The model under review builds one solid part; all positions refer to its coordinate system, in mm. A direction names the side the tool comes from. Coordinates: 2 decimals unless noted, no trailing zeros. Write each loop counter-clockwise with the first axis right and the second up, starting at its lowest first coordinate (ties: lowest second). Pieces come first, ordered by that corner, then holes. Notation, with made-up numbers: (50.5, 51) - (95.5, 51) arc R22 cw to (95.5, 68) - close; hole circle Ø7 at (63, 13.25). An arc over 180 degrees is marked (long way). Put each result on its own line as item: value.
from build123d import *

# Parameters (mm, degrees)
SKETCH1_W            = 688.1
SKETCH1_H            = 688.1
SKETCH1_W_2          = 650
SKETCH1_H_2          = 650
BOSS_EXTRUDE1_DEPTH  = 661.9
SKETCH3_W            = 100.2
SKETCH3_H            = 650
SKETCH3_W_2          = 38.6
CUT_EXTRUDE1_DEPTH   = 9.525
SKETCH4_W            = 100.2
SKETCH4_H            = 669.5
SKETCH4_W_2          = 38.6
SKETCH4_H_2          = 669.05
CUT_EXTRUDE3_DEPTH   = 9.525
SKETCH6_W            = 100.2
SKETCH6_H            = 669.5
SKETCH6_W_2          = 38.6
CUT_EXTRUDE4_DEPTH   = 9.525
CUT_EXTRUDE5_DEPTH   = 700
MIRROR6_COPY_1_DEPTH = 700


with BuildPart() as part:
    # Sketch1 → Boss-Extrude1 (new body)
    with BuildSketch(Plane(origin=(0, 0, 0), x_dir=(0, 0, -1), z_dir=(1, 0, 0))):
        with Locations((344.05, 344.05)):
            Rectangle(SKETCH1_W, SKETCH1_H)
        with Locations((344.05, 344.05)):
            Rectangle(SKETCH1_W_2, SKETCH1_H_2, mode=Mode.SUBTRACT)
    extrude(amount=BOSS_EXTRUDE1_DEPTH)

    # Sketch3 → Cut-Extrude1 (cut)
    with BuildSketch(Plane.XY.offset(-669.05)):
        with Locations((171.225, 344.05)):
            Rectangle(SKETCH3_W, SKETCH3_H)
        with Locations((361.75, 344.05)):
            Rectangle(SKETCH3_W_2, SKETCH3_H)
        with Locations((521.475, 344.05)):
            Rectangle(SKETCH3_W_2, SKETCH3_H)
    cut_extrude1 = extrude(amount=-CUT_EXTRUDE1_DEPTH, mode=Mode.SUBTRACT)

    # Mirror2: Cut-Extrude1 across plane
    add(cut_extrude1.mirror(Plane(origin=(0, 0, -344.05), x_dir=(1, 0, 0), z_dir=(0, 0, -1))), mode=Mode.SUBTRACT)

    # Sketch4 → Cut-Extrude3 (cut)
    with BuildSketch(Plane(origin=(0, 19.05, 0), x_dir=(1, 0, 0), z_dir=(0, 1, 0))):
        with Locations((171.225, 343.825)):
            Rectangle(SKETCH4_W, SKETCH4_H)
        with Locations((361.75, 343.825)):
            Rectangle(SKETCH4_W_2, SKETCH4_H)
        with Locations((521.475, 344.05)):
            Rectangle(SKETCH4_W_2, SKETCH4_H_2)
    cut_extrude3 = extrude(amount=-CUT_EXTRUDE3_DEPTH, mode=Mode.SUBTRACT)

    # Mirror4: Cut-Extrude3 across plane
    add(cut_extrude3.mirror(Plane.ZX.offset(344.05)), mode=Mode.SUBTRACT)

    # Sketch6 → Cut-Extrude4 (cut)
    with BuildSketch(Plane(origin=(0, 688.1, 0), x_dir=(1, 0, 0), z_dir=(0, 1, 0))):
        with Locations((171.225, 344.275)):
            Rectangle(SKETCH6_W, SKETCH6_H)
        with Locations((361.75, 343.825)):
            Rectangle(SKETCH6_W_2, SKETCH6_H)
        with Locations((521.475, 343.825)):
            Rectangle(SKETCH6_W_2, SKETCH6_H)
    extrude(amount=-CUT_EXTRUDE4_DEPTH, mode=Mode.SUBTRACT)

    # Sketch7 → Cut-Extrude5 (cut)
    with BuildSketch(Plane.ZY):
        Polygon((-19.05, 39.05), (-9.525, 39.05), (-9.525, 9.525), (-39.05, 9.525), (-39.05, 19.05), (-19.05, 19.05), align=None)
    cut_extrude5 = extrude(amount=-CUT_EXTRUDE5_DEPTH, mode=Mode.SUBTRACT)

    # Mirror5: Cut-Extrude5 across plane
    add(cut_extrude5.mirror(Plane(origin=(0, 0, -344.05), x_dir=(1, 0, 0), z_dir=(0, 0, -1))), mode=Mode.SUBTRACT)

    # Mirror6: Cut-Extrude5 across plane
    add(cut_extrude5.mirror(Plane.ZX.offset(344.05)), mode=Mode.SUBTRACT)

    # Mirror6 copy 1 sketch → Mirror6 copy 1 (cut)
    with BuildSketch(Plane(origin=(0, 688.1, -688.1), x_dir=(0, 0, -1), z_dir=(-1, 0, 0))):
        Polygon((-19.05, 39.05), (-9.525, 39.05), (-9.525, 9.525), (-39.05, 9.525), (-39.05, 19.05), (-19.05, 19.05), align=None)
    extrude(amount=-MIRROR6_COPY_1_DEPTH, mode=Mode.SUBTRACT)


solid = part.part
1. The part is to be moulded in two halves that separate along Z. For faces 1 (the flat face through (661.9, 14, -342)), 2 (the flat face through (540.775, 679, -339)), 3 (the flat face through (326, 339, -688.1)), say which applies: +Z half, -Z half, draft (parallel to the pull), parting line (faces both ways), or undercut.
Determined:
face 1: draft
face 2: undercut
face 3: -Z half
2. Machinability: for faces 4 (the flat face through (354, 367, -9.525)), 5 (the flat face through (121.125, 679, -340)), 6 (the flat face through (281, 340, -19.05)), which of the approach directions +Z, -Z, +X, -X, +Y, -Y give a long, thin tool a straight path to every point of the face, cutting with its end or side? Answer none if there is none.
Determined:
face 4: none
face 5: +Y
face 6: +X, -X
3. Consider section C-C on x = 285. State the section outline as (y, z) points (3 decimals), plus the area to 3 significant figures.
Determined:
outline: (0, -688.1) - (688.1, -688.1) - (688.1, 0) - (0, 0) - close; hole (9.525, -678.575) - (39.05, -678.575) - (39.05, -669.05) - (649.05, -669.05) - (649.05, -678.575) - (678.575, -678.575) - (678.575, -649.05) - (669.05, -649.05) - (669.05, -39.05) - (678.575, -39.05) - (678.575, -9.525) - (649.05, -9.525) - (649.05, -19.05) - (39.05, -19.05) - (39.05, -9.525) - (9.525, -9.525) - (9.525, -39.05) - (19.05, -39.05) - (19.05, -649.05) - (9.525, -649.05) - close
area: 49,100 mm^2
4. Consider section B-B on z = -342.5. Give the number of separate pieces and of enclosed holes in the cut face, plus the area to 3 significant figures.
Determined:
separate pieces: 5
enclosed holes: 0
area: 20,100 mm^2
5. To check wall thickness, follow probe 1 along Z at (x, y) = (325, 561); probe 2 along Z at (x, y) = (519.5, 646) (3 decimals); probe 3 along Y at (x, z) = (89.5, -547). State the ranges of each line that lie inside material, in increasing order.
Determined:
probe 1: z = -688.1 to -669.05, -19.05 to 0
probe 2: z = -688.1 to -678.575, -9.525 to 0
probe 3: y = 0 to 19.05, 669.05 to 688.1
